Design review of the part built by this model. Coordinates are the model's own, in mm. Face numbers are marked on the shaded views. Give positions to 0.01 mm unless a question says otherwise; leave off trailing zeros. Use a Markdown table: item, result. Add a question column.
(1) Add section A-A, the plane x = -45.1. State how many separate pieces and enclosed holes the cut face has, then the cut area to 3 significant figures.
(2) Draft analysis for pull direction Z (two halves, no side actions). For the marked faces 1 and 2, state which applies: pulls with the +Z half, pulls with the -Z half, needs draft (parallel to the pull), parting line crosses it, or undercut.
(3) For probe 1 along X at (y, z) = (5, 29.5); probe 2 along Z at (x, y) = (45.1, 4.55); probe 3 along Y at (x, z) = (-35.1, -29.75), list the stretches that pass through material, from the lowest coordinate up.
(4) Insertion check: pin 1 Ø5 at (x, y) = (4.5, 3) entering from -Z; pin 2 Ø0.9 at (x, y) = (36, 5) entering from -Z; pin 3 Ø1 at (y, z) = (9.5, 5) entering from -X; pin 4 Ø8 at (x, z) = (25.5, 6) entering from -Y. Each pin has a flat end and moves straight along its axis. Give the tip position at first contact, or say it passes through.
```python
from build123d import *

# Parameters (mm, degrees)
SKETCH_4_R          = 1.5
CUT_EXTRUDE_1_DEPTH = 20
SKETCH_5_R          = 1.5
CUT_EXTRUDE_2_DEPTH = 65.884590004
SKETCH3_W           = 30
SKETCH3_H           = 42
CUT_EXTRUDE1_DEPTH  = 65.884590004
CUT_EXTRUDE2_DEPTH  = 42


with BuildPart() as part:
    # Эскиз1 → По сечениям1 section 0
    with BuildSketch(Plane(origin=(0, 0, 0), x_dir=(1, 0, 0), z_dir=(0, 1, 0))):
        with BuildLine():
            Line((-50.1, -40), (50.1, -40))
            Line((50.1, -40), (50.1, 40))
            Line((50.1, 40), (-50.1, 40))
            Line((-50.1, 40), (-50.1, -40))
        make_face()
    # Эскиз2 → По сечениям1 section 1
    with BuildSketch(Plane(origin=(0, 10, 0), x_dir=(1, 0, 0), z_dir=(0, 1, 0))):
        with BuildLine():
            Line((40.1, -30), (40.1, 30))
            Line((40.1, 30), (-40.1, 30))
            Line((-40.1, 30), (-40.1, -30))
            Line((-40.1, -30), (40.1, -30))
        make_face()
    loft()

    # Эскиз4 → Вырез-Вытянуть1 (cut)
    with BuildSketch(Plane.XY.offset(40)):
        with Locations((-35.1, 5)):
            Circle(SKETCH_4_R)
        with Locations(Location((35.1, 5, 0), (0, 0, 270))):
            Circle(SKETCH_4_R)
    cut_extrude_1 = extrude(amount=-CUT_EXTRUDE_1_DEPTH, mode=Mode.SUBTRACT)

    # Зеркальное отражение1: Вырез-Вытянуть1 across plane
    add(cut_extrude_1.mirror(Plane.XY), mode=Mode.SUBTRACT)

    # Эскиз5 → Вырез-Вытянуть2 (cut, through all)
    with BuildSketch(Plane.XZ):
        with Locations(Location((-45.1, 15, 0), (0, 0, 270))):
            Circle(SKETCH_5_R)
        with Locations(Location((-45.1, -15, 0), (0, 0, 180))):
            Circle(SKETCH_5_R)
        with Locations(Location((45.1, -15, 0), (0, 0, 270))):
            Circle(SKETCH_5_R)
        with Locations((45.1, 15)):
            Circle(SKETCH_5_R)
    extrude(amount=-CUT_EXTRUDE_2_DEPTH, mode=Mode.SUBTRACT)

    # Cut-Loft1: read off the stored shape, not the designer's step
    # Cut-Loft1: loft between two sections, ruled curve by curve
    cut_loft1_from = [
        Edge.make_bspline([(-43.923484762, 2.8, 15.930490137), (-45.784465036, 2.8, 18.283520613), (-48.137495512, 2.8, 16.422540339), (-46.276515238, 2.8, 14.069509863), (-44.415534964, 2.8, 11.716479387), (-42.062504488, 2.8, 13.577459661), (-43.923484762, 2.8, 15.930490137)], [0, 0, 0, 0, 0.5, 0.5, 0.5, 1, 1, 1, 1], 3, [1, 0.333333333, 0.333333333, 1, 0.333333333, 0.333333333, 1]),
    ]
    cut_loft1_to = [
        Edge.make_bspline([(-43.881334244, 0, 18.066733405), (-50.014801053, 0, 20.504064917), (-52.452132565, 0, 14.370598107), (-46.318665756, 0, 11.933266595), (-40.185198947, 0, 9.495935083), (-37.747867435, 0, 15.629401893), (-43.881334244, 0, 18.066733405)], [0, 0, 0, 0, 0.5, 0.5, 0.5, 1, 1, 1, 1], 3, [1, 0.333333333, 0.333333333, 1, 0.333333333, 0.333333333, 1]),
    ]
    cut_loft1 = Solid(Shell([*[Face.make_surface_from_curves(cut_loft1_from[k], cut_loft1_to[k]) for k in range(1)], Face(Wire(cut_loft1_from)), Face(Wire(cut_loft1_to))]))
    add(cut_loft1, mode=Mode.SUBTRACT)

    # Mirror1: Cut-Loft1 across plane
    add(cut_loft1.mirror(Plane.XY), mode=Mode.SUBTRACT)

    # Mirror2: read off the stored shape, not the designer's step
    # Mirror2: loft between two sections, ruled curve by curve
    mirror2_from = [
        Edge.make_bspline([(43.923484762, 2.8, 15.930490137), (45.784465036, 2.8, 18.283520613), (48.137495512, 2.8, 16.422540339), (46.276515238, 2.8, 14.069509863), (44.415534964, 2.8, 11.716479387), (42.062504488, 2.8, 13.577459661), (43.923484762, 2.8, 15.930490137)], [0, 0, 0, 0, 0.5, 0.5, 0.5, 1, 1, 1, 1], 3, [1, 0.333333333, 0.333333333, 1, 0.333333333, 0.333333333, 1]),
    ]
    mirror2_to = [
        Edge.make_bspline([(43.881334244, 0, 18.066733405), (50.014801053, 0, 20.504064917), (52.452132565, 0, 14.370598107), (46.318665756, 0, 11.933266595), (40.185198947, 0, 9.495935083), (37.747867435, 0, 15.629401893), (43.881334244, 0, 18.066733405)], [0, 0, 0, 0, 0.5, 0.5, 0.5, 1, 1, 1, 1], 3, [1, 0.333333333, 0.333333333, 1, 0.333333333, 0.333333333, 1]),
    ]
    mirror2 = Solid(Shell([*[Face.make_surface_from_curves(mirror2_from[k], mirror2_to[k]) for k in range(1)], Face(Wire(mirror2_from)), Face(Wire(mirror2_to))]))
    add(mirror2, mode=Mode.SUBTRACT)

    # Mirror2 2: loft between two sections, ruled curve by curve
    mirror2_2_from = [
        Edge.make_bspline([(43.923484762, 2.8, -15.930490137), (45.784465036, 2.8, -18.283520613), (48.137495512, 2.8, -16.422540339), (46.276515238, 2.8, -14.069509863), (44.415534964, 2.8, -11.716479387), (42.062504488, 2.8, -13.577459661), (43.923484762, 2.8, -15.930490137)], [0, 0, 0, 0, 0.5, 0.5, 0.5, 1, 1, 1, 1], 3, [1, 0.333333333, 0.333333333, 1, 0.333333333, 0.333333333, 1]),
    ]
    mirror2_2_to = [
        Edge.make_bspline([(43.881334244, 0, -18.066733405), (50.014801053, 0, -20.504064917), (52.452132565, 0, -14.370598107), (46.318665756, 0, -11.933266595), (40.185198947, 0, -9.495935083), (37.747867435, 0, -15.629401893), (43.881334244, 0, -18.066733405)], [0, 0, 0, 0, 0.5, 0.5, 0.5, 1, 1, 1, 1], 3, [1, 0.333333333, 0.333333333, 1, 0.333333333, 0.333333333, 1]),
    ]
    mirror2_2 = Solid(Shell([*[Face.make_surface_from_curves(mirror2_2_from[k], mirror2_2_to[k]) for k in range(1)], Face(Wire(mirror2_2_from)), Face(Wire(mirror2_2_to))]))
    add(mirror2_2, mode=Mode.SUBTRACT)

    # Sketch3 → Cut-Extrude1 (cut, through all)
    with BuildSketch(Plane.XZ):
        with Locations((0, 2)):
            Rectangle(SKETCH3_W, SKETCH3_H)
    extrude(amount=-CUT_EXTRUDE1_DEPTH, mode=Mode.SUBTRACT)

    # Sketch4 → Cut-Extrude2 (cut)
    with BuildSketch(Plane.XY.offset(-19)):
        Polygon((-15, 8.8), (-17, 6.8), (-15, 4.8), align=None)
        Polygon((15, 4.8), (15, 8.8), (17, 6.8), align=None)
    extrude(amount=CUT_EXTRUDE2_DEPTH, mode=Mode.SUBTRACT)


solid = part.part
```
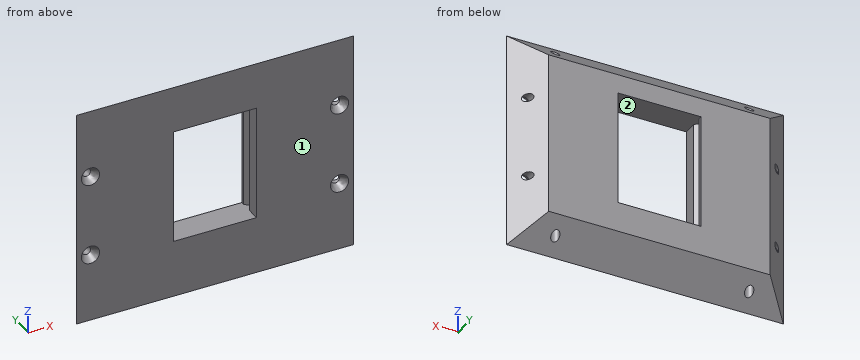
Established:
| question | item | result |
|---|---|---|
| 1 | separate pieces | 3 |
| 1 | enclosed holes | 0 |
| 1 | area | 335 mm^2 |
| 2 | face 1 | needs draft |
| 2 | face 2 | undercut |
| 3 | probe 1 | -45.1 to -36.6, -33.6 to 33.6, 36.6 to 45.1 |
| 3 | probe 2 | -35.45 to -16.5, -13.5 to 13.5, 16.5 to 35.45 |
| 3 | probe 3 | 0 to 3.5, 6.5 to 10 |
| 4 | pin 1 | z = -39.5 |
| 4 | pin 2 | z = -20 |
| 4 | pin 3 | x = -41.1 |
| 4 | pin 4 | y = 0 |
